Build history of the part. All positions in model axes, mm. Face numbers are marked on the shaded views. A direction names the side the tool comes from. Coordinates: 2 decimals unless noted, no trailing zeros. Loops run counter-clockwise (first coordinate to the right, second up) from the corner with the lowest first, then second, coordinate; pieces in that order, holes last.
(1) Slice it at C-C (z = -32). Give the cut face in (x, y), and give its area (3 significant figures).
(2) Wall check: L1, parallel to Z at x = 22.5, y = 566; L2, parallel to X at y = 570, z = -27.5; L3, parallel to Y at x = 0, z = -3. Give the ranges that are in metal, low to high.
(3) Two-plate mould, pull along Z, no slides. Class the marked faces 1, 2, 3 and 4: pulls with the +Z half, pulls with the -Z half, needs draft (parallel to the pull), parting line crosses it, or undercut.
(4) Flat gauge pins, fed straight in: P1, Ø3, axis at x = -22, z = 15, coming from the -Y side; P2, Ø11, axis at x = -3, z = 32, coming from the -Y side; P3, Ø15, axis at x = 2.5, z = -7.5, coming from the -Y side. Where does each tip first touch, or does it go through?
(5) Tool access for the marked faces 5, 6, 7 and 8: list every direction of +Z, -Z, +X, -X, +Y, -Y with a clear straight run to the whole face (end or side of a thin tool).
(6) Slice it at A-A (z = 8.5). Give the cut face in (x, y), and give its area (3 significant figures).
(7) Slice it at B-B (y = 541.5). Give the cut face in (x, z), and give its area (3 significant figures).
(8) Slice it at D-D (y = 415). Give the cut face in (x, z).
from build123d import *

# Parameters (mm, degrees)
BOSS_EXTRUDE1_DEPTH      = 40
BOSS_EXTRUDE1_DEPTH_BACK = 40
SKETCH1_R                = 10
CUT_EXTRUDE2_DEPTH       = 20
CUT_EXTRUDE2_DEPTH_BACK  = 20
CUT_EXTRUDE4_START       = -20
CUT_EXTRUDE4_DEPTH       = 20
CUT_EXTRUDE6_START       = -20
CUT_EXTRUDE6_DEPTH       = 20
FILLET3_R                = 5
SHELL1_START             = -15
SHELL1_OUTLINE_R         = 15
SHELL1_DEPTH             = 30
SHELL1_START_2           = -35
SHELL1_2_OUTLINE_W       = 60.710678118
SHELL1_2_OUTLINE_H       = 50
SHELL1_2_DEPTH           = 70
SHELL1_3_OUTLINE_R       = 15
SHELL1_3_DEPTH           = 10
SHELL1_START_3           = 25
SHELL1_4_OUTLINE_R       = 15
SHELL1_4_DEPTH           = 10
SHELL1_START_4           = -30.355339059
SHELL1_5_DEPTH           = 60.710678118


with BuildPart() as part:
    # Sketch1 → Boss-Extrude1 (new, two sides: drawn at the far end of the back side and taken through both)
    with BuildSketch(Plane.XY.offset(-BOSS_EXTRUDE1_DEPTH_BACK)):
        with BuildLine():
            Line((-35.355339059, 370), (-35.355339059, 570))
            ThreePointArc((-35.355339059, 570), (0, 605.355339059), (35.355339059, 570))
            Line((35.355339059, 570), (35.355339059, 370))
            ThreePointArc((35.355339059, 370), (0, 334.644660941), (-35.355339059, 370))
        make_face()
        with Locations(Location((0, 370, 0), (0, 0, 180))):
            Circle(SKETCH1_R, mode=Mode.SUBTRACT)
        with Locations(Location((0, 570, 0), (0, 0, 180))):
            Circle(SKETCH1_R, mode=Mode.SUBTRACT)
    extrude(amount=BOSS_EXTRUDE1_DEPTH + BOSS_EXTRUDE1_DEPTH_BACK)

    # Sketch2 → Cut-Extrude2 (cut, two sides: drawn at the far end of the back side and taken through both)
    with BuildSketch(Plane.XY.offset(-CUT_EXTRUDE2_DEPTH_BACK)):
        with BuildLine():
            Line((-35.355339059, 530), (35.355339059, 530))
            Line((35.355339059, 530), (35.355339059, 570))
            ThreePointArc((35.355339059, 570), (0, 605.355339059), (-35.355339059, 570))
            Line((-35.355339059, 570), (-35.355339059, 530))
        make_face()
    extrude(amount=CUT_EXTRUDE2_DEPTH + CUT_EXTRUDE2_DEPTH_BACK, mode=Mode.SUBTRACT)

    # Sketch3 → Cut-Extrude4 (cut)
    with BuildSketch(Plane.XY.offset(40).offset(CUT_EXTRUDE4_START)):
        with BuildLine():
            Line((-35.355339059, 370), (-35.355339059, 470))
            Line((-35.355339059, 470), (35.355339059, 470))
            Line((35.355339059, 470), (35.355339059, 370))
            ThreePointArc((35.355339059, 370), (0, 334.644660941), (-35.355339059, 370))
        make_face()
    extrude(amount=CUT_EXTRUDE4_DEPTH, mode=Mode.SUBTRACT)

    # Sketch5 → Cut-Extrude6 (cut)
    with BuildSketch(Plane(origin=(0, 0, -40), x_dir=(-1, 0, 0), z_dir=(0, 0, -1)).offset(CUT_EXTRUDE6_START)):
        with BuildLine():
            Line((-35.355339059, 370), (-35.355339059, 470))
            Line((-35.355339059, 470), (35.355339059, 470))
            Line((35.355339059, 470), (35.355339059, 370))
            ThreePointArc((35.355339059, 370), (0, 334.644660941), (-35.355339059, 370))
        make_face()
    extrude(amount=CUT_EXTRUDE6_DEPTH, mode=Mode.SUBTRACT)

    # Fillet3
    fillet3_edges = [part.edges().sort_by_distance(p)[0] for p in [
        (0, 530, -20),
        (0, 530, 20),
        (0, 470, 40),
        (0, 470, 20),
        (0, 470, -40),
        (0, 470, -20),
    ]]
    fillet(fillet3_edges, radius=FILLET3_R)

    # Shell1: read off the stored shape, not the designer's step
    # Shell1 outline → Shell1 (cut)
    with BuildSketch(Plane.XY.offset(SHELL1_START)):
        with BuildLine():
            ThreePointArc((-30.355339059, 370), (0, 339.644660941), (30.355339059, 370))
            Line((30.355339059, 370), (30.355339059, 525))
            Line((30.355339059, 525), (-30.355339059, 525))
            Line((-30.355339059, 525), (-30.355339059, 370))
        make_face()
        with Locations((0, 370)):
            Circle(SHELL1_OUTLINE_R, mode=Mode.SUBTRACT)
    extrude(amount=SHELL1_DEPTH, mode=Mode.SUBTRACT)

    # Shell1 2 outline → Shell1 2 (cut)
    with BuildSketch(Plane.XY.offset(SHELL1_START_2)):
        with Locations((0, 500)):
            Rectangle(SHELL1_2_OUTLINE_W, SHELL1_2_OUTLINE_H)
    extrude(amount=SHELL1_2_DEPTH, mode=Mode.SUBTRACT)

    # Shell1 3 outline → Shell1 3 (cut)
    with BuildSketch(Plane.XY.offset(SHELL1_START_2)):
        with BuildLine():
            Line((-30.355339059, 525), (30.355339059, 525))
            Line((30.355339059, 525), (30.355339059, 570))
            ThreePointArc((30.355339059, 570), (0, 600.355339059), (-30.355339059, 570))
            Line((-30.355339059, 570), (-30.355339059, 525))
        make_face()
        with Locations((0, 570)):
            Circle(SHELL1_3_OUTLINE_R, mode=Mode.SUBTRACT)
    extrude(amount=SHELL1_3_DEPTH, mode=Mode.SUBTRACT)

    # Shell1 4 outline → Shell1 4 (cut)
    with BuildSketch(Plane.XY.offset(SHELL1_START_3)):
        with BuildLine():
            Line((-30.355339059, 525), (30.355339059, 525))
            Line((30.355339059, 525), (30.355339059, 570))
            ThreePointArc((30.355339059, 570), (0, 600.355339059), (-30.355339059, 570))
            Line((-30.355339059, 570), (-30.355339059, 525))
        make_face()
        with Locations((0, 570)):
            Circle(SHELL1_4_OUTLINE_R, mode=Mode.SUBTRACT)
    extrude(amount=SHELL1_4_DEPTH, mode=Mode.SUBTRACT)

    # Shell1 5 outline → Shell1 5 (cut)
    with BuildSketch(Plane.YZ.offset(SHELL1_START_4)):
        with BuildLine():
            ThreePointArc((535, -25), (527.928932188, -22.071067812), (525, -15))
            Line((525, -15), (525, -25))
            Line((525, -25), (535, -25))
        make_face()
        with BuildLine():
            ThreePointArc((525, 15), (527.928932188, 22.071067812), (535, 25))
            Line((535, 25), (525, 25))
            Line((525, 25), (525, 15))
        make_face()
        with BuildLine():
            ThreePointArc((475, 25), (472.071067812, 17.928932188), (465, 15))
            Line((465, 15), (475, 15))
            Line((475, 15), (475, 25))
        make_face()
        with BuildLine():
            Line((475, -15), (465, -15))
            ThreePointArc((465, -15), (472.071067812, -17.928932188), (475, -25))
            Line((475, -25), (475, -15))
        make_face()
    extrude(amount=SHELL1_5_DEPTH, mode=Mode.SUBTRACT)


solid = part.part
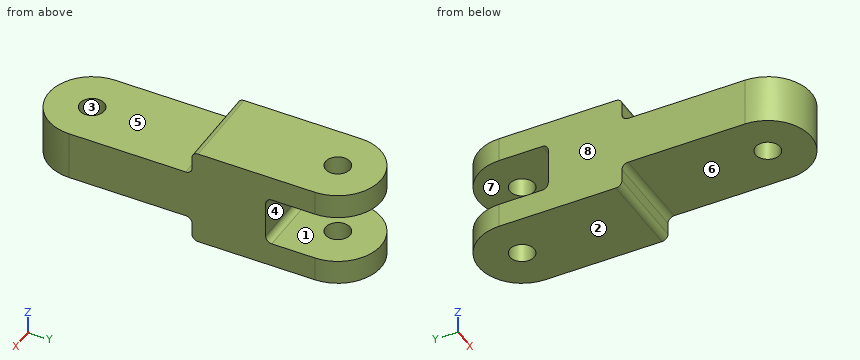
Response values:
1. outline: (-35.36, 470) - (35.36, 470) - (35.36, 570) arc R35.36 ccw to (-35.36, 570) - close; circle Ø30 at (0, 570); hole (-30.36, 475) - (30.36, 475) - (30.36, 570) arc R30.36 ccw to (-30.36, 570) - close; hole circle Ø20 at (0, 570)
1. area: 2,210 mm2
2. L1: z = -40 to -35, -25 to -20, 20 to 25, 35 to 40
2. L2: x = -35.36 to -30.36, -15 to -10, 10 to 15, 30.36 to 35.36
2. L3: y = 334.64 to 339.64, 355 to 360, 380 to 385, 525 to 530
3. face 1: undercut
3. face 2: pulls with the -Z half
3. face 3: needs draft
3. face 4: undercut
4. P1: stops at y = 341.19
4. P2: stops at y = 470
4. P3: stops at y = 334.64
5. face 5: +Z, +X, -X, -Y
5. face 6: -Z, +X, -X, -Y
5. face 7: +X, -X, +Y
5. face 8: +Z, -Z, -X, +Y, -Y
6. outline: (-35.36, 370) arc R35.36 ccw to (35.36, 370) - (35.36, 530) - (-35.36, 530) - close; circle Ø30 at (0, 370); hole (-30.36, 370) arc R30.36 ccw to (30.36, 370) - (30.36, 525) - (-30.36, 525) - close; hole circle Ø20 at (0, 370)
6. area: 2,810 mm2
7. outline: (-35.36, -40) - (35.36, -40) - (35.36, -20) - (-35.36, -20) - close; (-35.36, 20) - (35.36, 20) - (35.36, 40) - (-35.36, 40) - close; hole (-30.36, -35) - (30.36, -35) - (30.36, -25) - (-30.36, -25) - close; hole (-30.36, 25) - (30.36, 25) - (30.36, 35) - (-30.36, 35) - close
7. area: 1,610 mm2
8. outline: (-35.36, -20) - (35.36, -20) - (35.36, 20) - (-35.36, 20) - close; hole (-30.36, -15) - (30.36, -15) - (30.36, 15) - (-30.36, 15) - close
